Geometry: final body of the model. Coordinates: model frame, mm. Face numbers are marked on the shaded views. A direction names the side the tool comes from. Give positions to 0.01 mm unless a question says otherwise; leave off trailing zeros. Write each loop counter-clockwise with the first axis right and the second up, starting at its lowest first coordinate (ties: lowest second). Pieces come first, ordered by that corner, then holes. Notation, with made-up numbers: (-36, 63.5) - (-13, 63.5) arc R21 cw to (-13, 75.5) - close; hole circle Ø6 at (-10.5, 60). An arc over 180 degrees is marked (long way). Return JSON: item names as keys, results as strings.
from build123d import *

# Parameters (mm, degrees)
BOSS_EXTRUDE1_DEPTH = 1
BOSS_EXTRUDE2_DEPTH = 6
CUT_EXTRUDE1_DEPTH  = 4
CUT_EXTRUDE2_DEPTH  = 4
SKETCH6_W           = 1
SKETCH6_H           = 2
CUT_EXTRUDE3_DEPTH  = 4
BOSS_EXTRUDE3_DEPTH = 4
SKETCH8_W           = 2
SKETCH8_H           = 4
CUT_EXTRUDE4_DEPTH  = 4
BOSS_EXTRUDE4_DEPTH = 1
SKETCH14_W          = 4.502969787
SKETCH14_H          = 1
CUT_EXTRUDE6_DEPTH  = 4
SKETCH11_W          = 3
SKETCH11_H          = 2
CUT_EXTRUDE5_DEPTH  = 2
BOSS_EXTRUDE5_DEPTH = 5
SKETCH16_W          = 1
SKETCH16_H          = 2
CUT_EXTRUDE7_DEPTH  = 3


with BuildPart() as part:
    # Sketch2 → Boss-Extrude1 (new body)
    with BuildSketch(Plane.XY):
        Polygon((0, 0), (0, 3), (5, 8), (8, 8), (8, 0), align=None)
    extrude(amount=BOSS_EXTRUDE1_DEPTH)

    # Sketch3 → Boss-Extrude2 (add)
    with BuildSketch(Plane.XY.offset(1)):
        Polygon((0, 0), (0, 3), (2, 5), (3.00380266, 5), (3.00380266, 3), (3.00380266, 0), align=None)
    extrude(amount=BOSS_EXTRUDE2_DEPTH)

    # Sketch4 → Cut-Extrude1 (cut)
    with BuildSketch(Plane.ZY):
        Polygon((3, 5), (7, 1), (7, 5), align=None)
    extrude(amount=-CUT_EXTRUDE1_DEPTH, mode=Mode.SUBTRACT)

    # Sketch5 → Cut-Extrude2 (cut)
    with BuildSketch(Plane(origin=(0, 5, 0), x_dir=(1, 0, 0), z_dir=(0, 1, 0))):
        Polygon((1, -4), (1, -3), (0, -3), (0, -3.75), (0, -7), (2, -7), (2, -4), align=None)
    extrude(amount=-CUT_EXTRUDE2_DEPTH, mode=Mode.SUBTRACT)

    # Sketch6 → Cut-Extrude3 (cut)
    with BuildSketch(Plane(origin=(0, 1, 0), x_dir=(1, 0, 0), z_dir=(0, 1, 0))):
        with Locations((0.5, -6)):
            Rectangle(SKETCH6_W, SKETCH6_H)
    extrude(amount=-CUT_EXTRUDE3_DEPTH, mode=Mode.SUBTRACT)

    # Sketch7 → Boss-Extrude3 (add)
    with BuildSketch(Plane(origin=(3.00380266, 0, 0), x_dir=(0, 0, -1), z_dir=(1, 0, 0))):
        Polygon((-7, 0), (-7, 1), (-4, 4), (-1, 4), (-1, 0), align=None)
    extrude(amount=BOSS_EXTRUDE3_DEPTH)

    # Sketch8 → Cut-Extrude4 (cut)
    with BuildSketch(Plane(origin=(0, 4, 0), x_dir=(1, 0, 0), z_dir=(0, 1, 0))):
        with Locations((5.00380266, -5)):
            Rectangle(SKETCH8_W, SKETCH8_H)
    extrude(amount=-CUT_EXTRUDE4_DEPTH, mode=Mode.SUBTRACT)

    # Sketch9 → Boss-Extrude4 (add)
    with BuildSketch(Plane(origin=(7.00380266, 0, 0), x_dir=(0, 0, -1), z_dir=(1, 0, 0))):
        Polygon((-7, 0), (-1, 0), (-1, 8), (-5, 8), (-7, 4), align=None)
    extrude(amount=BOSS_EXTRUDE4_DEPTH)

    # Sketch14 → Cut-Extrude6 (cut)
    with BuildSketch(Plane(origin=(3.00380266, 0, 0), x_dir=(0, 0, -1), z_dir=(1, 0, 0))):
        with Locations((-3.251484894, 3.5)):
            Rectangle(SKETCH14_W, SKETCH14_H)
    extrude(amount=CUT_EXTRUDE6_DEPTH, mode=Mode.SUBTRACT)

    # Sketch11 → Cut-Extrude5 (cut)
    with BuildSketch(Plane(origin=(8.00380266, 0, 0), x_dir=(0, 0, -1), z_dir=(1, 0, 0))):
        with Locations((-3.5, 5)):
            Rectangle(SKETCH11_W, SKETCH11_H)
    extrude(amount=-CUT_EXTRUDE5_DEPTH, mode=Mode.SUBTRACT)

    # Sketch15 → Boss-Extrude5 (add)
    with BuildSketch(Plane(origin=(0, 3, 0), x_dir=(1, 0, 0), z_dir=(0, 1, 0))):
        Polygon((7.00380266, -3), (5.00380266, -1), (7.00380266, -1), align=None)
    extrude(amount=BOSS_EXTRUDE5_DEPTH)

    # Sketch16 → Cut-Extrude7 (cut)
    with BuildSketch(Plane(origin=(7.00380266, 0, 0), x_dir=(0, 0, -1), z_dir=(1, 0, 0))):
        with Locations((-2.5, 5)):
            Rectangle(SKETCH16_W, SKETCH16_H)
    extrude(amount=-CUT_EXTRUDE7_DEPTH, mode=Mode.SUBTRACT)


solid = part.part
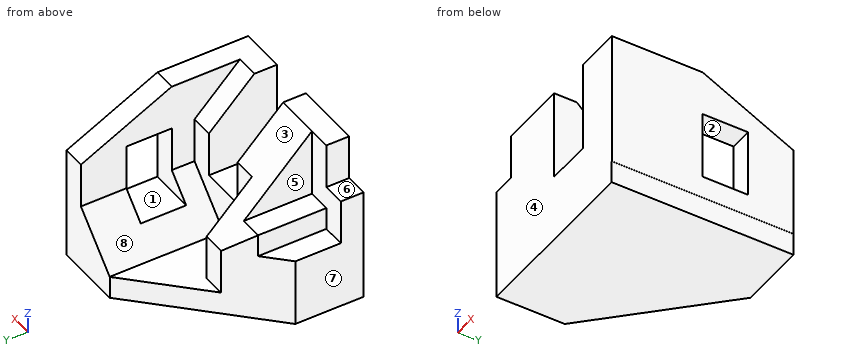
Q1. Section query A-A, the plane z = 6.5. Return the cut outline in (x, y).
Answer key:
{"outline": "(1, 0) - (4, 0) - (4, 1.5) - (2, 1.5) - (2, 1) - (1, 1) - close; (6, 0) - (8, 0) - (8, 5) - (7, 5) - (7, 1.5) - (6, 1.5) - close"}
Q2. Material intervals for probe 1 along X at (y, z) = (5, 6.25); probe 2 along Y at (x, z) = (5, 1.25); probe 3 along Z at (x, y) = (3.75, 6), sorted ascending. Write a range as [from, to].
Answer key:
{"probe 1": "x = [7, 8]", "probe 2": "y = [0, 3]", "probe 3": "z = [0, 1]"}
Q3. Section query D-D, the plane x = 7.25. Return the cut outline in (y, z), plus the area to 3 significant figures.
Answer key:
{"outline": "(0, 0) - (8, 0) - (8, 5) - (4, 7) - (0, 7) - close; hole (4, 2) - (6, 2) - (6, 5) - (4, 5) - close", "area": "46.0 mm^2"}
Q4. Pin query (flat end, axial travel): P1, Ø0.5, axis at x = 7.5, y = 4.5, coming from the -Z side; P2, Ø0.5, axis at y = 5, z = 0.5, coming from the +X side; P3, Ø3, axis at x = 3, y = 3, coming from the +Z side; P4, Ø0.5, axis at y = 3, z = 3.5, coming from the -X side. Return the tip coordinate at first contact, or that it passes through.
Answer key:
{"P1": "stops at z = 0", "P2": "stops at x = 8", "P3": "stops at z = 6.5", "P4": "stops at x = 1"}
Q5. Section query B-B, the plane x = 1.5. Return the cut outline in (y, z).
Answer key:
{"outline": "(0, 0) - (4.5, 0) - (4.5, 3.5) - (4, 4) - (1, 4) - (1, 7) - (0, 7) - close"}
Q6. Set-up query: the marked faces 5, 6, 7 and 8. Return all of +Z, -Z, +X, -X, +Y, -Y with unobstructed straight access to the full face (end or side cutting, diameter ignored); none if empty.
Answer key:
{"face 5": "+Z, -X, +Y", "face 6": "+Z, -X, +Y, -Y", "face 7": "+Z, -Z, -X, +Y, -Y", "face 8": "+Z, +Y"}
Q7. Mould query, pull axis Y, two halves, no side actions, for the marked faces 1, 2, 3 and 4. Classes: pulls with the +Y half, pulls with the -Y half, needs draft (parallel to the pull), parting line crosses it, or undercut.
Answer key:
{"face 1": "undercut", "face 2": "undercut", "face 3": "pulls with the +Y half", "face 4": "pulls with the -Y half"}
